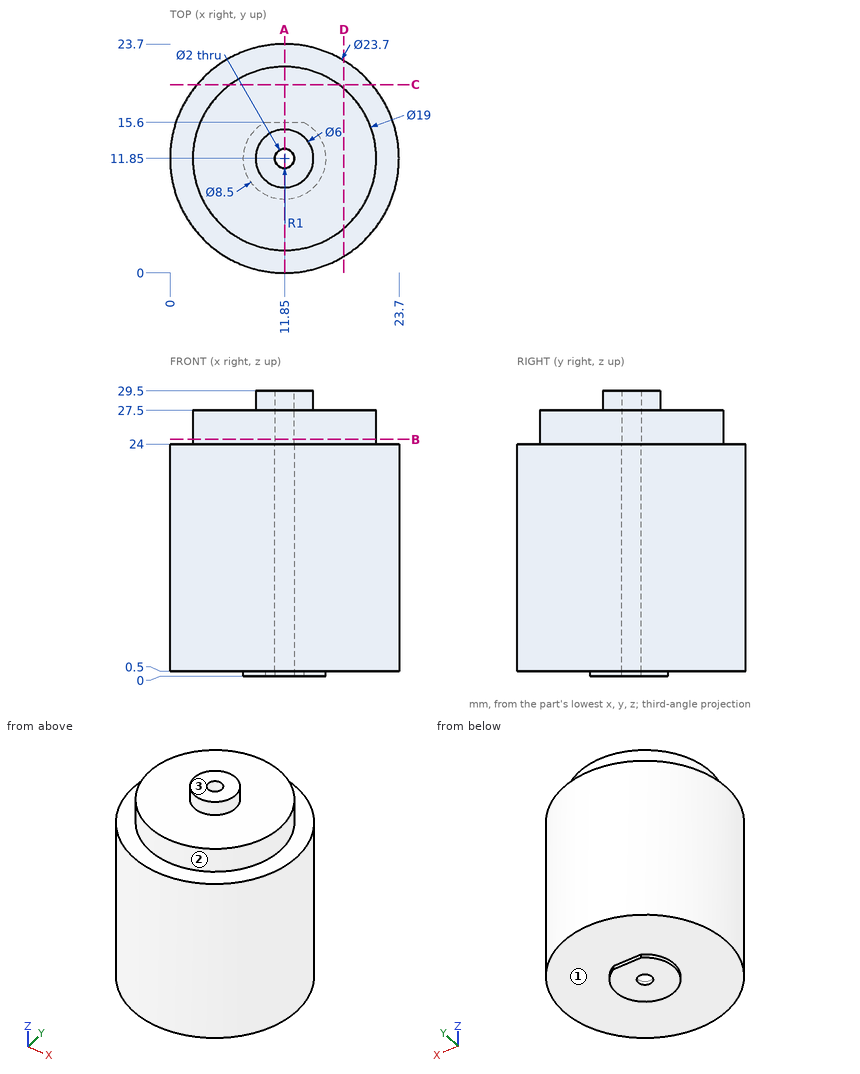
Source: three-view drawing plus pictorial views. Frame: mm from the lowest corner of the part. A direction names the side the tool comes from. Coordinates: 2 decimals unless noted, no trailing zeros. Order: outer loops, then holes, each group sorted by start corner. A loop starts at its lowest first (then second) coordinate and runs counter-clockwise, first axis right, second up. Notation, with made-up numbers: (62.5, 27.5) -> (119.5, 27.5) arc R23 cw to (119.5, 46.5) -> close; hole circle Ø1 at (-19, -3). An arc over 180 degrees is marked (long way). Write item = value, one per line.
(1) Cut plane C-C on y = 19.5. Return loops of the section in (x, z).
Solved:
outline = (2.8, 0.5) -> (20.9, 0.5) -> (20.9, 24) -> (17.48, 24) -> (17.48, 27.5) -> (6.22, 27.5) -> (6.22, 24) -> (2.8, 24) -> close
(2) Pin query (flat end, axial travel): pin 1 Ø1 at (x, y) = (15, 8) entering from +Z; pin 2 Ø2 at (y, z) = (6, 15) entering from +X; pin 3 Ø6 at (x, z) = (4.5, 3.5) entering from +Y. Return the tip coordinate at first contact, or that it passes through.
Solved:
pin_1 = 27.5
pin_2 = 22.66
pin_3 = 22.87
(3) Line query: line 1 (Y direction, x = 11.85, z = 13.5); line 2 (Z direction, x = 7.5, y = 13.5); line 3 (X direction, y = 11, z = 19.5). Output: solid intervals per line, ascending.
Solved:
line_1 = 0 to 10.85, 12.85 to 23.7
line_2 = 0.5 to 27.5
line_3 = 0.03 to 11.32, 12.38 to 23.67
(4) Cut plane A-A on x = 11.85. Return loops of the section in (y, z), plus the area to 3 significant figures.
Solved:
outline = (0, 0.5) -> (7.6, 0.5) -> (7.6, 0) -> (10.85, 0) -> (10.85, 29.5) -> (8.85, 29.5) -> (8.85, 27.5) -> (2.35, 27.5) -> (2.35, 24) -> (0, 24) -> close; (12.85, 0) -> (15.6, 0) -> (15.6, 0.5) -> (23.7, 0.5) -> (23.7, 24) -> (21.35, 24) -> (21.35, 27.5) -> (14.85, 27.5) -> (14.85, 29.5) -> (12.85, 29.5) -> close
area = 580 mm²
(5) Cut plane B-B on z = 24.5. Return loops of the section in (x, y).
Solved:
outline = circle Ø19 at (11.85, 11.85); hole circle Ø2 at (11.85, 11.85)
(6) Cut plane D-D on x = 18. Return loops of the section in (y, z), plus the area to 3 significant figures.
Solved:
outline = (1.72, 0.5) -> (21.98, 0.5) -> (21.98, 24) -> (19.09, 24) -> (19.09, 27.5) -> (4.61, 27.5) -> (4.61, 24) -> (1.72, 24) -> close
area = 527 mm²
(7) Access query for the marked faces 1, 2 and 3. Directions: +Z, -Z, +X, -X, +Y, -Y. A direction counts if a zero-diameter tool reaches every point of the face in a straight line with its end or side. Return the directions, or none.
Solved:
face_1 = -Z
face_2 = +Z
face_3 = +Z, +X, -X, +Y, -Y
